Here's how the part is built. I have some questions about the finished solid (model axes, mm). Round coordinates to 2 decimals unless told otherwise and drop trailing zeros. Write each loop counter-clockwise with the first axis right and the second up, starting at its lowest first coordinate (ties: lowest second). Pieces come first, ordered by that corner, then holes. Notation, with made-up numbers: (38, -7.75) - (58, -7.75) arc R23 ccw to (58, 14.25) - close; hole circle Ø8 at (-24.75, 42.25). An arc over 180 degrees is marked (long way). Write item = value, one per line. Start each with the question number.
Item 1: If we section it at B-B (z = -5): Please give me the cut outline in (x, y).
Item 2: If we section it at D-D (z = 5.75): Please give me the cut outline in (x, y), and give its area (3 significant figures).
Item 3: If we section it at A-A (x = 0): Please give me the cut outline in (y, z), and give its area (3 significant figures).
Item 4: If we section it at C-C (y = 0): Please give me the cut outline in (x, z).
Item 5: If I drill on line 1 along Z through (x, y) = (0, -0.15); line 2 along Z through (x, y) = (0.4, -0.25); line 3 along X through (y, z) = (0.1, -5), over which ranges is the centre line in solid material (lowest first)? Write a range as [from, to].
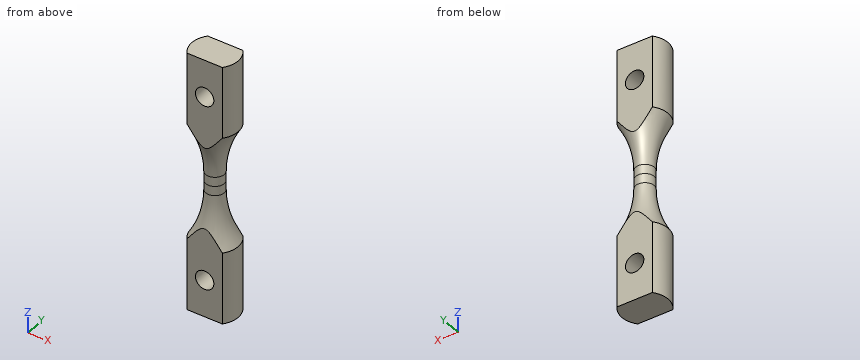
```python
from build123d import *

# Parameters (mm, degrees)
F2_W     = 1.25
F2_H     = 7
F3_DEPTH = 0.8
F4_R     = 0.5
F5_DEPTH = 12.5


# Not quite as in the source:
# - a feature names something its author has since deleted; it is built from what else it names


with BuildPart() as f1:
    # F0 (on Front) → F1 (revolve)
    with BuildSketch(Plane.XZ):
        with BuildLine():
            Line((1.25, 7), (0, 7))
            Line((0, 7), (0, 0))
            Line((0, 0), (0, -7))
            Line((0, -7), (1.25, -7))
            Line((1.25, -7), (1.25, -3.1339134382))
            ThreePointArc((1.25, -3.1339134382), (0.6911539846, -1.8693063938), (0.5, -0.5))
            Line((0.5, -0.5), (0.5, 0.5))
            ThreePointArc((0.5, 0.5), (0.6911539846, 1.8693063938), (1.25, 3.1339134382))
            Line((1.25, 3.1339134382), (1.25, 7))
        make_face()
    revolve(axis=Axis((0, 0, 3.5), (0, 0, -1)))

    # F2 (on Front) → F3 (intersect, symmetric)
    with BuildSketch(Plane.XZ):
        with Locations((0.625, 3.5)):
            Rectangle(F2_W, F2_H)
        with Locations((-0.625, 3.5)):
            Rectangle(F2_W, F2_H)
    extrude(amount=F3_DEPTH, both=True, mode=Mode.INTERSECT)

    # F4 (on Front) → F5 (cut, symmetric)
    with BuildSketch(Plane.XZ):
        with Locations((0, 5)):
            Circle(F4_R)
    extrude(amount=F5_DEPTH, both=True, mode=Mode.SUBTRACT)

    # F6: F1 across plane


with BuildPart() as f1_1:
    add(f1.part)
    add(f1.part.mirror(Plane.XY))


solid = f1_1.part
```
Reply:
q1.outline = (-0.96, -0.8) - (-0.5, -0.8) - (-0.5, 0.8) - (-0.96, 0.8) arc R1.25 ccw to start; (0.5, -0.8) - (0.96, -0.8) arc R1.25 ccw to (0.96, 0.8) - (0.5, 0.8) - close
q2.outline = (-0.96, -0.8) - (0.96, -0.8) arc R1.25 ccw to (0.96, 0.8) - (-0.96, 0.8) arc R1.25 ccw to start
q2.area = 3.71 mm2
q3.outline = (-0.8, -7) - (0.8, -7) - (0.8, -5.5) - (-0.8, -5.5) - close; (-0.8, -4.5) - (0.8, -4.5) - (0.8, -2.21) arc R5 cw to (0.5, -0.5) - (0.5, 0.5) arc R5 cw to (0.8, 2.21) - (0.8, 4.5) - (-0.8, 4.5) - (-0.8, 2.21) arc R5 cw to (-0.5, 0.5) - (-0.5, -0.5) arc R5 cw to (-0.8, -2.21) - close; (-0.8, 5.5) - (0.8, 5.5) - (0.8, 7) - (-0.8, 7) - close
q3.area = 17.2 mm2
q4.outline = (-1.25, -7) - (1.25, -7) - (1.25, -3.13) arc R5 cw to (0.5, -0.5) - (0.5, 0.5) arc R5 cw to (1.25, 3.13) - (1.25, 7) - (-1.25, 7) - (-1.25, 3.13) arc R5 cw to (-0.5, 0.5) - (-0.5, -0.5) arc R5 cw to (-1.25, -3.13) - close; hole circle Ø1 at (0, -5); hole circle Ø1 at (0, 5)
q5.line_1 = [-7, -5.5], [-4.5, 4.5], [5.5, 7]
q5.line_2 = [-7, -5.3], [-4.7, 4.7], [5.3, 7]
q5.line_3 = [-1.25, -0.5], [0.5, 1.25]
